Input: dimensioned drawing with shaded views. Units: mm. Origin: part minimum x, y, z. A direction names the side the tool comes from. Coordinates: 2 decimals unless noted, no trailing zeros. Write each loop counter-clockwise with the first axis right and the second up, starting at its lowest first coordinate (ties: lowest second). Pieces come first, ordered by that corner, then holes. Notation, with made-up numbers: M 2.5,63.25 L 42.5,63.25 A20 cw 42.5,94.25 Z; hole C 48.25,82.25 d11. An arc over 180 degrees is marked long. Write each question's results on one line, items separated by ' | '. Start each with the question number.
1. Section query D-D, the plane x = 12. Output: boundary loops of the cut face in (y, z), and give its area (3 significant figures).
2. Section query A-A, the plane y = 1.75. Output: boundary loops of the cut face in (x, z).
3. First-contact query: pin 1 (9 mm diameter, centred on x = 54, z = 67.5, fed in from -Y). Flat tip, straight axial feed; report the tip coordinate or a pass-through.
4. Pull-direction query (Z, two-part tool) for the marked faces 1, 2, 3 and 4; classes: +Z half, -Z half, draft (parallel to the pull), parting line (faces both ways), or undercut.
5. Set-up query: the marked faces 5 and 6. Return all of +Z, -Z, +X, -X, +Y, -Y with unobstructed straight access to the full face (end or side cutting, diameter ignored); none if empty.
6. Section query B-B, the plane z = 27. Output: boundary loops of the cut face in (x, y), and give its area (3 significant figures).
7. Ray query, probe 1 along X at (y, z) = (4.25, 62.75); probe 2 along Y at (x, z) = (135, 25); probe 3 along X at (y, z) = (6.75, 62.75). Return the intervals inside material, ascending.
8. Section query C-C, the plane x = 38. Output: boundary loops of the cut face in (y, z).
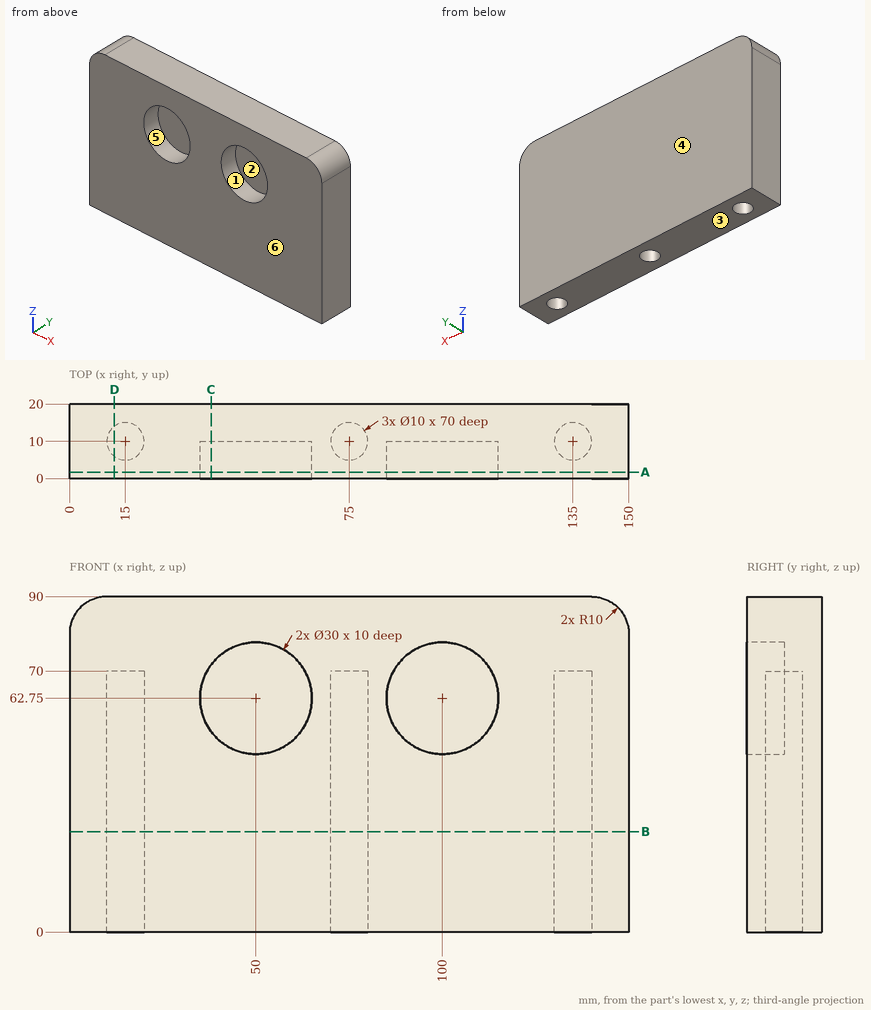
Answer:
1) outline: M 0,0 L 6,0 L 6,70 L 14,70 L 14,0 L 20,0 L 20,90 L 0,90 Z | area: 1,240 mm^2
2) outline: M 0,0 L 150,0 L 150,80 A10 ccw 140,90 L 10,90 A10 ccw 0,80 Z; hole C 50,62.75 d30; hole C 100,62.75 d30
3) pin 1: y = 10
4) face 1: undercut | face 2: undercut | face 3: -Z half | face 4: draft
5) face 5: -Y | face 6: +Z, -Z, +X, -X, -Y
6) outline: M 0,0 L 150,0 L 150,20 L 0,20 Z; hole C 15,10 d10; hole C 75,10 d10; hole C 135,10 d10 | area: 2,760 mm^2
7) probe 1: 0 to 35, 65 to 85, 115 to 150 | probe 2: 0 to 5, 15 to 20 | probe 3: 0 to 11.2, 18.8 to 35, 65 to 71.2, 78.8 to 85, 115 to 131.2, 138.8 to 150
8) outline: M 0,0 L 20,0 L 20,90 L 0,90 L 0,71.75 L 10,71.75 L 10,53.75 L 0,53.75 Z
